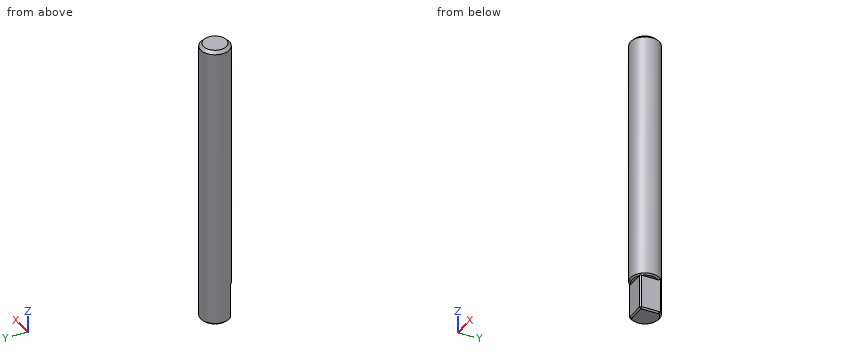
from build123d import *

# Parameters (mm, degrees)
F0_R         = 5
F1_DEPTH     = 100
F3_DEPTH     = 12
F4_SIZE      = 1
F5_SIZE      = 0.5
F6_T2_ANGLE  = 209.430321651
F6_T6_ANGLE  = 59.8137801049
F6_T12_ANGLE = 149.7566863334
F6_T18_ANGLE = 149.7566863334
F6_T25_ANGLE = 149.7566863334
F6_T31_ANGLE = 149.7566863334
F6_T38_ANGLE = 149.7566863334
F6_T45_ANGLE = 149.7566863334


# Not quite as in the source:
# - a fillet or chamfer that OpenCascade refuses, or shapes differently, is made with other operations: its cross-section is extruded or revolved along the edge and cut away or added


with BuildPart() as f1:
    # F0 (on Top) → F1 (new body)
    with BuildSketch(Plane.XY):
        Circle(F0_R)
    extrude(amount=F1_DEPTH)

    # F2 (on face) → F3 (cut)
    with BuildSketch(Plane(origin=(0, 0, 0), x_dir=(1, 0, 0), z_dir=(0, 0, -1))):
        with BuildLine():
            Line((-3.5, 3.5), (3.5, 3.5))
            Line((3.5, 3.5), (3.5, -3.5))
            Line((3.5, -3.5), (3.5307399131, -3.5403214072))
            ThreePointArc((3.5307399131, -3.5403214072), (4.6181002352, -1.9165464297), (5, 0))
            ThreePointArc((5, 0), (1.9130662834, 4.6195429855), (-3.5360709581, 3.5349967722))
            Line((-3.5360709581, 3.5349967722), (-3.5, 3.5))
        make_face()
    extrude(amount=-F3_DEPTH, mode=Mode.SUBTRACT)

    # F4
    f4_edges = [f1.edges().sort_by_distance(p)[0] for p in [
        (-5, 0, 100),
    ]]
    chamfer(f4_edges, length=F4_SIZE)

    # F5
    f5_edges = [f1.edges().sort_by_distance(p)[0] for p in [
        (0, -3.5, 0),
        (3.5, 0, 0),
        (3.5, -3.5, 6),
    ]]
    chamfer(f5_edges, length=F5_SIZE)

    # F6: chamfer of 0.5 on 3 edges, made by hand

    # F6_s1 → F6_t2 (revolve, cut)
    with BuildSketch(Plane(origin=(0, 0, 0), x_dir=(0, 0, 1), z_dir=(0.5048185175, -0.8632255003, 0))):
        Polygon((0.5, -5), (0, -4.5), (0, -5), align=None)
    revolve(axis=Axis((0, 0, 0), (0, 0, 1)), revolution_arc=F6_T2_ANGLE, mode=Mode.SUBTRACT)


with BuildPart() as f6_tool4:
    # F6_s5 → F6_t6 (revolve)
    with BuildSketch(Plane(origin=(0, 0, 0), x_dir=(0, 0, 1), z_dir=(-0.8643957574, 0.5028120669, 0))):
        Polygon((12, 4.5), (12.5, 5), (12, 5), align=None)
    revolve(axis=Axis((0, 0, 12), (0, 0, -1)), revolution_arc=F6_T6_ANGLE)

    split(bisect_by=Plane.YZ.offset(3.5), keep=Keep.TOP)

    split(bisect_by=Plane(origin=(0.5259878903, -0.4009984555, 0), x_dir=(0, 0, 1), z_dir=(0.7952525516, -0.6062783018, 0)), keep=Keep.TOP)


with BuildPart() as f1_1:
    add(f1.part)

    # F6_t3: cut F6_tool4
    add(f6_tool4.part, mode=Mode.SUBTRACT)


with BuildPart() as f6_tool10:
    # F6_s11 → F6_t12 (revolve)
    with BuildSketch(Plane.XZ):
        Polygon((4.5, 12), (5, 12.5), (5, 12), align=None)
    revolve(axis=Axis((0, 0, 12), (0, 0, -1)), revolution_arc=F6_T12_ANGLE)

    split(bisect_by=Plane(origin=(3.25, -3.25, 0), x_dir=(0, 0, 1), z_dir=(-0.7071067812, 0.7071067812, 0)), keep=Keep.TOP)

    split(bisect_by=Plane.YZ.offset(3.5), keep=Keep.TOP)


with BuildPart() as f1_2:
    add(f1_1.part)

    # F6_t9: cut F6_tool10
    add(f6_tool10.part, mode=Mode.SUBTRACT)


with BuildPart() as f6_tool16:
    # F6_s17 → F6_t18 (revolve)
    with BuildSketch(Plane.XZ):
        Polygon((4.5, 12), (5, 12.5), (5, 12), align=None)
    revolve(axis=Axis((0, 0, 12), (0, 0, -1)), revolution_arc=F6_T18_ANGLE)

    split(bisect_by=Plane.XZ.offset(3.5), keep=Keep.BOTTOM)

    split(bisect_by=Plane(origin=(3.25, -3.25, 0), x_dir=(0, 0, 1), z_dir=(0.7071067812, -0.7071067812, 0)), keep=Keep.TOP)

    split(bisect_by=Plane.YZ.offset(3.5), keep=Keep.TOP)


with BuildPart() as f1_3:
    add(f1_2.part)

    # F6_t15: cut F6_tool16
    add(f6_tool16.part, mode=Mode.SUBTRACT)


with BuildPart() as f6_tool23:
    # F6_s24 → F6_t25 (revolve)
    with BuildSketch(Plane.XZ):
        Polygon((4.5, 12), (5, 12.5), (5, 12), align=None)
    revolve(axis=Axis((0, 0, 12), (0, 0, -1)), revolution_arc=F6_T25_ANGLE)

    split(bisect_by=Plane.XZ.offset(3.5), keep=Keep.TOP)

    split(bisect_by=Plane.YZ.offset(3.5), keep=Keep.TOP)


with BuildPart() as f1_4:
    add(f1_3.part)

    # F6_t22: cut F6_tool23
    add(f6_tool23.part, mode=Mode.SUBTRACT)


with BuildPart() as f6_tool29:
    # F6_s30 → F6_t31 (revolve)
    with BuildSketch(Plane.XZ):
        Polygon((4.5, 12), (5, 12.5), (5, 12), align=None)
    revolve(axis=Axis((0, 0, 12), (0, 0, -1)), revolution_arc=F6_T31_ANGLE)

    split(bisect_by=Plane.XZ.offset(3.5), keep=Keep.BOTTOM)

    split(bisect_by=Plane(origin=(3.25, -3.25, 0), x_dir=(0, 0, 1), z_dir=(0.7071067812, -0.7071067812, 0)), keep=Keep.TOP)

    split(bisect_by=Plane.YZ.offset(3.5), keep=Keep.BOTTOM)


with BuildPart() as f1_5:
    add(f1_4.part)

    # F6_t28: cut F6_tool29
    add(f6_tool29.part, mode=Mode.SUBTRACT)


with BuildPart() as f6_tool36:
    # F6_s37 → F6_t38 (revolve)
    with BuildSketch(Plane.XZ):
        Polygon((4.5, 12), (5, 12.5), (5, 12), align=None)
    revolve(axis=Axis((0, 0, 12), (0, 0, -1)), revolution_arc=F6_T38_ANGLE)

    split(bisect_by=Plane.XZ.offset(3.5), keep=Keep.TOP)

    split(bisect_by=Plane(origin=(3.25, -3.25, 0), x_dir=(0, 0, 1), z_dir=(-0.7071067812, 0.7071067812, 0)), keep=Keep.TOP)

    split(bisect_by=Plane(origin=(0.0520908408, -0.0536897095, 0), x_dir=(0, 0, 1), z_dir=(0.6963393518, -0.7177126913, 0)), keep=Keep.TOP)


with BuildPart() as f1_6:
    add(f1_5.part)

    # F6_t35: cut F6_tool36
    add(f6_tool36.part, mode=Mode.SUBTRACT)


with BuildPart() as f6_tool43:
    # F6_s44 → F6_t45 (revolve)
    with BuildSketch(Plane.XZ):
        Polygon((4.5, 12), (5, 12.5), (5, 12), align=None)
    revolve(axis=Axis((0, 0, 12), (0, 0, -1)), revolution_arc=F6_T45_ANGLE)

    split(bisect_by=Plane.XZ.offset(3.5), keep=Keep.TOP)

    split(bisect_by=Plane(origin=(3.25, -3.25, 0), x_dir=(0, 0, 1), z_dir=(0.7071067812, -0.7071067812, 0)), keep=Keep.TOP)

    split(bisect_by=Plane.YZ.offset(3.5), keep=Keep.BOTTOM)


with BuildPart() as f1_7:
    add(f1_6.part)

    # F6_t42: cut F6_tool43
    add(f6_tool43.part, mode=Mode.SUBTRACT)


solid = f1_7.part
Verification items for the finished model (mm, model axes). Coordinates: 2 decimals unless noted, no trailing zeros. Loops run counter-clockwise (first coordinate to the right, second up) from the corner with the lowest first, then second, coordinate; pieces in that order, holes last. Notation, with made-up numbers: (72, 63) -> (128, 63) arc R12 cw to (128, 73) -> close; hole circle Ø1 at (50, 4). An arc over 180 degrees is marked (long way). Answer as a JSON object with one key per item and string values. Group by question number.
Item 1: Scan lines: probe 1 along Y at (x, z) = (3, 92); probe 2 along X at (y, z) = (-4, 18.5). Record each from-to range of solid material in increasing order.
Item 2: Sectioned sample at C-C on z = 18. Record the boundary of the cut face in (x, y), plus the area to 3 significant figures.
Item 3: Sectioned sample at A-A on y = 0. Record the boundary of the cut face in (x, z).
Item 4: Depth check by flat-ended pin: pin 1 (5 mm diameter, centred on y = -1, z = 5, fed in from +X); pin 2 (2 mm diameter, centred on y = -2.5, z = 30.5, fed in from -X); pin 3 (3.5 mm diameter, centred on x = -1.5, z = 8, fed in from -Y). Enter the tip coordinate at first touch or a pass-through.
Item 5: Sectioned sample at B-B on x = 0. Record the boundary of the cut face in (y, z), plus the area to 3 significant figures.
Evaluation:
{
 "1": {"probe 1": "y = -4 to 4", "probe 2": "x = -3 to 3"},
 "2": {"outline": "circle Ø10 at (0, 0)", "area": "78.5 mm²"},
 "3": {"outline": "(-5, 0.5) -> (-4.5, 0) -> (3, 0) -> (3.5, 0.5) -> (3.5, 12) -> (4.5, 12) -> (5, 12.5) -> (5, 99) -> (4, 100) -> (-4, 100) -> (-5, 99) -> close"},
 "4": {"pin 1": "stops at x = 3.5", "pin 2": "stops at x = -4.77", "pin 3": "stops at y = -3.5"},
 "5": {"outline": "(-5, 12.5) -> (-4.5, 12) -> (-3.5, 12) -> (-3.5, 0.5) -> (-3, 0) -> (4.5, 0) -> (5, 0.5) -> (5, 99) -> (4, 100) -> (-4, 100) -> (-5, 99) -> close", "area": "981 mm²"}
}
